from build123d import *

# Parameters (mm, degrees)
F0_W     = 625.475
F0_H     = 257.175
F0_R     = 1.905
F0_W_2   = 581.025
F0_H_2   = 212.725
F1_DEPTH = 1.524


with BuildPart() as f1:
    # F0 (on Top) → F1 (new body)
    with BuildSketch(Plane.XY):
        with Locations((300.0375, 106.3625)):
            Rectangle(F0_W, F0_H)
        Circle(F0_R, mode=Mode.SUBTRACT)
        with Locations((600.075, 0)):
            Circle(F0_R, mode=Mode.SUBTRACT)
        with Locations((300.0375, 106.3625)):
            Rectangle(F0_W_2, F0_H_2, mode=Mode.SUBTRACT)
        with Locations((0, 212.725)):
            Circle(F0_R, mode=Mode.SUBTRACT)
        with Locations((600.075, 212.725)):
            Circle(F0_R, mode=Mode.SUBTRACT)
    extrude(amount=F1_DEPTH)


solid = f1.part
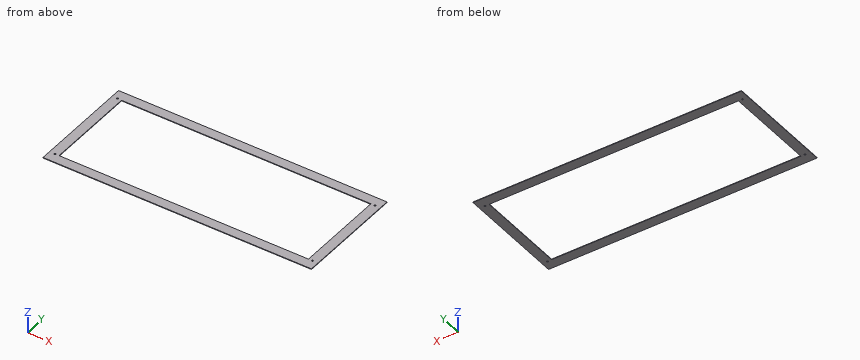
Model file for the job. Use its own axes, mm. Give positions to 0.01 mm unless a question says otherwise; leave off trailing zeros. Order: outer loops, then holes, each group sorted by start corner. A loop starts at its lowest first (then second) coordinate and runs counter-clockwise, first axis right, second up. Notation, with made-up numbers: (-35, -4.5) -> (-17, -4.5) arc R22 ccw to (-17, 28.5) -> close; hole circle Ø1 at (-7, 14). An arc over 180 degrees is marked (long way). Use CSV: the item, a comma, the result in double quotes.
1. Band-saw the part on C-C, the plane x = 401. Give the cut face in (y, z) (3 decimals).
Outcome:
outline,"(-22.225, 0) -> (0, 0) -> (0, 1.524) -> (-22.225, 1.524) -> close; (212.725, 0) -> (234.95, 0) -> (234.95, 1.524) -> (212.725, 1.524) -> close"
2. Drop a flat-ended pin along its axis: pin 1 (3 mm diameter, centred on x = 0, y = 212.725, fed in from -Z). Give the stop position or say it passes through.
Outcome:
pin 1,"through"
3. Band-saw the part on B-B, the plane z = 0.75. Give the cut face in (x, y) (3 decimals), then the cut area to 3 significant figures.
Outcome:
outline,"(-12.7, -22.225) -> (612.775, -22.225) -> (612.775, 234.95) -> (-12.7, 234.95) -> close; hole circle Ø3.81 at (0, 0); hole circle Ø3.81 at (0, 212.725); hole (9.525, 0) -> (590.55, 0) -> (590.55, 212.725) -> (9.525, 212.725) -> close; hole circle Ø3.81 at (600.075, 0); hole circle Ø3.81 at (600.075, 212.725)"
area,"37,200 mm²"
4. Band-saw the part on A-A, the plane y = 114.5. Give the cut face in (x, z) (3 decimals), then the cut area to 3 significant figures.
Outcome:
outline,"(-12.7, 0) -> (9.525, 0) -> (9.525, 1.524) -> (-12.7, 1.524) -> close; (590.55, 0) -> (612.775, 0) -> (612.775, 1.524) -> (590.55, 1.524) -> close"
area,"67.7 mm²"
5. Drill centre lines: line 1 along Y through (x, z) = (0, 0.6) (3 decimals); line 2 along X through (y, z) = (104.5, 0.7) (3 decimals); line 3 along Y through (x, z) = (415.5, 1.1) (3 decimals). Where is each one in solid material? Low to high. Write a range as from..to.
Outcome:
line 1,"-22.225..-1.905, 1.905..210.82, 214.63..234.95"
line 2,"-12.7..9.525, 590.55..612.775"
line 3,"-22.225..0, 212.725..234.95"
